The model under review builds one solid part; all positions refer to its coordinate system, in mm. A direction names the side the tool comes from. Round coordinates to 2 decimals unless told otherwise and drop trailing zeros. Order: outer loops, then holes, each group sorted by start corner. A loop starts at its lowest first (then second) coordinate and runs counter-clockwise, first axis right, second up. Notation, with made-up numbers: (-9.75, 8) -> (44.25, 8) arc R14 cw to (44.25, 30) -> close; hole circle Ø10 at (-0.75, 1.25). An arc over 180 degrees is marked (long way). Put each result on its own line as item: value. Start each with the question number.
Autodesk Inventor part; units mm, degrees
sketch "Boceto1" plane through (0, 0, 0) normal (0, 0, 1) x (1, 0, 0)
  line L0 (-16, 11.5) -> (16, 11.5)
  line L1 (16, 11.5) -> (16, -11.5)
  line L2 (16, -11.5) -> (-16, -11.5)
  line L3 (-16, -11.5) -> (-16, 11.5)
  point P0 (0, 0)
  point P1 (16, 0)
  point P2 (0, 11.5)
  dimension "d0" = 32
  dimension "d1" = 23
extrude "Extrusión1" add sketch "Boceto1" along normal blind 34.25
fillet "Empalme1" radius 2 4 edges at (16, -11.5, 17.125) (16, 11.5, 17.125) (-16, 11.5, 17.125) (-16, -11.5, 17.125)
sketch "Boceto2" plane through (16, -9.5, 0) normal (1, 0, 0) x (0, 0, -1)
  line L0 (-34.25, 0) -> (-34.25, 19)
  line L1 (-34.25, 2.918) -> (-20.45, 2.918)
  line L2 (-20.45, 2.918) -> (-16.6504, 9.5)
  line L3 (-16.6504, 9.5) -> (-20.45, 16.082)
  line L4 (-20.45, 16.082) -> (-34.25, 16.082)
  line L5 (-34.25, 2.918) -> (-34.25, 16.082)
  point P0 (0, 9.5)
  point P1 (-34.25, 9.5)
  dimension "d5" = 13.8
  dimension "d6" = 7.6
  dimension "d7" = 13.164
extrude "Extrusión2" cut sketch "Boceto2" against normal blind 3.19
sketch "Boceto3" plane through (12.81, -9.5, 0) normal (1, 0, 0) x (0, 0, -1)
  line L0 (-20.45, 2.918) -> (-34.25, 2.918)
  line L1 (-16.6504, 9.5) -> (-20.45, 2.918)
  line L2 (-20.45, 16.082) -> (-16.6504, 9.5)
  line L3 (-34.25, 16.082) -> (-20.45, 16.082)
  line L4 (-34.25, 2.918) -> (-34.25, 16.082)
  line L5 (-34.25, 5.0035) -> (-24.25, 5.0035)
  arc A0 (-24.25, 5.0035) -> (-24.25, 13.9965) centre (-24.25, 9.5) ccw
  line L6 (-24.25, 13.9965) -> (-34.25, 13.9965)
  line L7 (-34.25, 2.918) -> (-34.25, 16.082)
  line L8 (-34.25, 5.0035) -> (-34.25, 13.9965)
  point P0 (0, 9.5)
  point P1 (-34.25, 9.5)
  dimension "d10" = 10
  dimension "d11" = 8.993
extrude "Extrusión3" cut sketch "Boceto3" against normal blind 2.9 contours L4 L6 A0 L5
sketch "Boceto4" plane through (-16, -9.5, 0) normal (-1, 0, 0) x (0, 0, 1)
  line L0 (34.25, 16.082) -> (20.45, 16.082)
  line L1 (20.45, 16.082) -> (16.6504, 9.5)
  line L2 (16.6504, 9.5) -> (20.45, 2.918)
  line L3 (20.45, 2.918) -> (34.25, 2.918)
  line L4 (34.25, 16.082) -> (34.25, 2.918)
  line L5 (34.25, 0) -> (34.25, 2.918)
  point P0 (0, 9.5)
extrude "Extrusión4" cut sketch "Boceto4" against normal blind 23.71
sketch "Boceto5" plane through (7.71, -9.5, 0) normal (-1, 0, 0) x (0, 0, 1)
  line L0 (34.25, 17.7) -> (24.25, 17.7)
  arc A0 (24.25, 17.7) -> (24.25, 1.3) centre (24.25, 9.5) ccw
  line L1 (24.25, 1.3) -> (34.25, 1.3)
  line L2 (20.45, 2.918) -> (34.25, 2.918)
  line L3 (34.25, 5.0035) -> (34.25, 13.9965)
  line L4 (34.25, 17.7) -> (34.25, 1.3)
  line L5 (34.25, 0) -> (34.25, 2.918)
  point P0 (0, 9.5)
  point P1 (34.25, 9.5)
  dimension "d16" = 10
  dimension "d17" = 16.4
extrude "Extrusión5" cut sketch "Boceto5" against normal up to surface (2.2 mm away)
sketch "Boceto6" plane through (0, 0, 0) normal (0, 0, -1) x (-1, 0, 0)
  line L0 (16, 0) -> (-7.71, 0)
  circle A0 centre (5, 0) radius 1.89
  circle A1 centre (-5, 0) radius 1.89
  line L1 (16, -9.5) -> (16, 9.5)
  point P0 (0, 0)
  dimension "d20" = 3.78
  dimension "d21" = 3.78
  dimension "d22" = 10
  dimension "d23" = 11
extrude "Extrusión6" cut sketch "Boceto6" against normal blind 7.21
sketch "Boceto7" plane through (-5, 0, 7.21) normal (0, 0, -1) x (-1, 0, 0)
  circle A0 centre (0, 0) radius 1.89
  circle A1 centre (-10, 0) radius 1.89
  line L0 (3.245, -1.8735) -> (0, -3.747)
  line L1 (0, -3.747) -> (-3.245, -1.8735)
  line L2 (-3.245, -1.8735) -> (-3.245, 1.8735)
  line L3 (-3.245, 1.8735) -> (0, 3.747)
  line L4 (0, 3.747) -> (3.245, 1.8735)
  line L5 (3.245, 1.8735) -> (3.245, -1.8735)
  line L6 (-6.755, -1.8735) -> (-10, -3.747)
  line L7 (-10, -3.747) -> (-13.245, -1.8735)
  line L8 (-13.245, -1.8735) -> (-13.245, 1.8735)
  line L9 (-13.245, 1.8735) -> (-10, 3.747)
  line L10 (-10, 3.747) -> (-6.755, 1.8735)
  line L11 (-6.755, 1.8735) -> (-6.755, -1.8735)
  point P0 (-5, 0)
  dimension "d26" = 3.747
  dimension "d27" = 3.747
extrude "Extrusión7" cut sketch "Boceto7" against normal through all contours A0 | A1 | L0 L1 L2 L3 L4 L5 | L6 L7 L8 L9 L10 L11
ref_plane "Plano de trabajo1" through (0, -9.5, 0) normal (-1, 0, 0) x (0, 0, 1)
Q1. Take a section at D-D on y = -5.5. Give the boundary of the cut face in (x, z), and give its area (3 significant figures).
Q2. Clearance check with flat-ended pins moving along their axes: pin 1 Ø1.5 at (x, y) = (-3.5, -8) entering from -Z; pin 2 Ø8 at (x, y) = (-2.5, -1) entering from +Z; pin 3 Ø4.5 at (x, y) = (-5, 0) entering from +Z; pin 4 Ø10.5 at (y, z) = (0, 26) entering from +X. State where each tip first meets the part, or that it passes through.
Q3. Take a section at B-B on x = -6. Give the boundary of the cut face in (y, z), and give its area (3 significant figures).
Q4. Draft analysis for pull direction X (two halves, no side actions). For faces 4 (the face through (8.245, 0, 12)), 5 (the face through (-16, 0, 13)), 6 (the face through (0, 11.5, 17)), 7 (the face through (4, -2, 7.21)), state which applies: +X half, -X half, draft (parallel to the pull), parting line (faces both ways), or undercut.
Q5. Wall thickness on probe 1 along X at (y, z) = (0, 5.5); probe 2 along Y at (x, z) = (-5, 3.75); probe 3 along Y at (x, z) = (2.5, 24.5): over which ranges is each line inside the solid? List them lowest first. Write a range as [from, to].
Q6. Take a section at A-A on z = 8.5. Give the boundary of the cut face in (x, y) (1 decimal).
Q7. For faces 1 (the face through (11, -4.496, 29)), 2 (the face through (-4, -6.582, 27)), 3 (the face through (-1.755, 0, 12)), list the 3-axis set-ups (+Z, -Z, +X, -X, +Y, -Y) from which the entire face can be reached by the end or side of a thin tool; tool diameter is ignored.
Q8. Take a section at C-C on x = -10.5. Give the boundary of the cut face in (y, z).
Calculated:
1. outline: (-16, 0) -> (16, 0) -> (16, 19.83) -> (12.81, 19.83) -> (12.81, 34.25) -> (9.91, 34.25) -> (9.91, 18.17) -> (7.71, 18.17) -> (7.71, 19.83) -> (-16, 19.83) -> close
1. area: 673 mm²
2. pin 1: stops at z = 0
2. pin 2: stops at z = 19.54
2. pin 3: stops at z = 7.21
2. pin 4: stops at x = 12.81
3. outline: (-11.5, 0) -> (-1.6, 0) -> (-1.6, 7.21) -> (-3.17, 7.21) -> (-3.17, 18.48) -> (-6.58, 20.45) -> (-6.58, 34.25) -> (-11.5, 34.25) -> close; (1.6, 0) -> (11.5, 0) -> (11.5, 34.25) -> (6.58, 34.25) -> (6.58, 20.45) -> (3.17, 18.48) -> (3.17, 7.21) -> (1.6, 7.21) -> close
3. area: 492 mm²
4. face 4: undercut
4. face 5: -X half
4. face 6: draft
4. face 7: undercut
5. probe 1: x = [-16, -6.89], [-3.11, 3.11], [6.89, 16]
5. probe 2: y = [-11.5, -1.89], [1.89, 11.5]
5. probe 3: y = [-11.5, -6.58], [6.58, 11.5]
6. outline: (-16, -9.5) arc R2 ccw to (-14, -11.5) -> (14, -11.5) arc R2 ccw to (16, -9.5) -> (16, 9.5) arc R2 ccw to (14, 11.5) -> (-14, 11.5) arc R2 ccw to (-16, 9.5) -> close; hole (-8.2, -1.9) -> (-5, -3.7) -> (-1.8, -1.9) -> (-1.8, 1.9) -> (-5, 3.7) -> (-8.2, 1.9) -> close; hole (1.8, -1.9) -> (5, -3.7) -> (8.2, -1.9) -> (8.2, 1.9) -> (5, 3.7) -> (1.8, 1.9) -> close
7. face 1: +Z, +X, -X
7. face 2: +Z, -X
7. face 3: +Z
8. outline: (-11.5, 0) -> (11.5, 0) -> (11.5, 34.25) -> (6.58, 34.25) -> (6.58, 20.45) -> (0, 16.65) -> (-6.58, 20.45) -> (-6.58, 34.25) -> (-11.5, 34.25) -> close
